Could you check a few things on this model? Use its own coordinates, in mm. A direction names the side the tool comes from. Round coordinates to 2 decimals unless told otherwise and drop trailing zeros. Write each loop counter-clockwise with the first axis right and the second up, starting at its lowest first coordinate (ties: lowest second). Pieces come first, ordered by that corner, then holes. Notation, with made-up numbers: (-30.5, -14.5) -> (28.5, -14.5) arc R15 ccw to (28.5, 14.5) -> close; hole circle Ø2 at (26, 66). An arc over 180 degrees is marked (long way). Answer in a Markdown table with one row per item.
from build123d import *

# Parameters (mm, degrees)
BOSS_EXTRUDE1_DEPTH = 70
CHAMFER1_SIZE       = 2


with BuildPart() as part:
    # Sketch1 → Boss-Extrude1 (new body)
    with BuildSketch(Plane(origin=(0, 0, 0), x_dir=(0, 0, -1), z_dir=(1, 0, 0))):
        Polygon((-7.2, 6.018181818), (7.527272727, 6.018181818), (7.527272727, -10.381818182), (7.527272727, -18.981818182), (3.218181818, -18.981818182), (3.218181818, -7.981818182), (3.218181818, 2.018181818), (-2.781818182, 2.018181818), (-2.781818182, -7.981818182), (-7.2, -7.981818182), align=None)
    extrude(amount=BOSS_EXTRUDE1_DEPTH)

    # Chamfer1
    chamfer1_edges = [part.edges().sort_by_distance(p)[0] for p in [
        (35, -7.981818182, 7.2),
    ]]
    chamfer(chamfer1_edges, length=CHAMFER1_SIZE)


solid = part.part
1) Please list where these lines run through material, in increasing order: line 1 (Z direction, x = 15.5, y = -0.25); line 2 (Z direction, x = 4, y = -7.75); line 3 (Y direction, x = 54, z = 0.25).
Findings:
| item | result |
|---|---|
| line 1 | z = -7.53 to -3.22, 2.78 to 7.2 |
| line 2 | z = -7.53 to -3.22, 2.78 to 5.43 |
| line 3 | y = 2.02 to 6.02 |
2) Imagine slicing it at D-D, the plane y = -12.75. Please give me the cut outline in (x, z).
Findings:
| item | result |
|---|---|
| outline | (0, -7.53) -> (70, -7.53) -> (70, -3.22) -> (0, -3.22) -> close |
3) Imagine slicing it at B-B, the plane x = 42. Please give me the cut outline in (y, z), plus the area to 3 significant figures.
Findings:
| item | result |
|---|---|
| outline | (-18.98, -7.53) -> (6.02, -7.53) -> (6.02, 7.2) -> (-5.98, 7.2) -> (-7.98, 5.2) -> (-7.98, 2.78) -> (2.02, 2.78) -> (2.02, -3.22) -> (-18.98, -3.22) -> close |
| area | 192 mm^2 |
4) For pin 1 (3 mm diameter, centred on x = 20, z = -0.5, fed in from -Y); pin 2 (1 mm diameter, centred on x = 54, y = -7.5, fed in from +Z); pin 3 (6.5 mm diameter, centred on x = 19, y = -9.5, fed in from +Z), each with a flat end and sliding along its axis, tell me the tip position at first contact or that it passes through.
Findings:
| item | result |
|---|---|
| pin 1 | stops at y = 2.02 |
| pin 2 | stops at z = 6.18 |
| pin 3 | stops at z = 6.93 |
5) Imagine slicing it at C-C, the plane z = -1.75. Please give me the cut outline in (x, y).
Findings:
| item | result |
|---|---|
| outline | (0, 2.02) -> (70, 2.02) -> (70, 6.02) -> (0, 6.02) -> close |
6) Thinking about a two-plate mould opening in Z: for faces 4 (the face through (34.51, -6.97, 6.21)), 5 (the face through (35, -7, -7.527)), 6 (the face through (35, 2.018, 0)), which applies, +Z half, -Z half, draft (parallel to the pull), parting line (faces both ways), or undercut?
Findings:
| item | result |
|---|---|
| face 4 | +Z half |
| face 5 | -Z half |
| face 6 | undercut |
7) Imagine slicing it at A-A, the plane y = -4.25. Please give me the cut outline in (x, z), plus the area to 3 significant figures.
Findings:
| item | result |
|---|---|
| outline | (0, -7.53) -> (70, -7.53) -> (70, -3.22) -> (0, -3.22) -> close; (0, 2.78) -> (70, 2.78) -> (70, 7.2) -> (0, 7.2) -> close |
| area | 611 mm^2 |
8) For faces 1 (the face through (0, -4, -4)), 2 (the face through (35, -7.982, 4)), 3 (the face through (35, -3, 2.782)), which set-ups out of +Z, -Z, +X, -X, +Y, -Y let a thin tool reach every point of the face, with its end or its side?
Findings:
| item | result |
|---|---|
| face 1 | +Z, -Z, -X, +Y, -Y |
| face 2 | +Z, +X, -X, -Y |
| face 3 | +X, -X, -Y |
